from build123d import *

# Parameters (mm, degrees)
F0_W     = 64.5160431693
F0_H     = 21.2102837178
F1_DEPTH = 25.4
F3_DEPTH = 51.816
F5_DEPTH = 78.486
F6_DEPTH = 43.18


with BuildPart() as f1:
    # F0 (on Top) → F1 (new body)
    with BuildSketch(Plane.XY):
        with Locations((-13.5457146427, -10.1202105203)):
            Rectangle(F0_W, F0_H)
        with Locations((-13.5457146427, -31.3304942381)):
            Rectangle(F0_W, F0_H)
        Polygon((-56.0653362274, -41.935636097), (-45.8037362274, -41.935636097), (-45.8037362274, -20.7253523792), (-45.8037362274, 0.4849313386), (-56.0653362274, 0.4849313386), (-56.0653362274, -20.7253523792), align=None)
    extrude(amount=F1_DEPTH)

    # F2 (on face) → F3 (cut)
    with BuildSketch(Plane.XZ.offset(41.935636097)):
        with BuildLine():
            ThreePointArc((-44.145979319, 1.0321285638), (-44.1486688564, 1.034928695), (-44.1513573992, 1.0377297813))
            Line((-44.1513573992, 1.0377297813), (-45.9468774498, 1.1715529611))
            Line((-45.9468774498, 1.1715529611), (-44.145979319, 1.0321285638))
        make_face()
        with BuildLine():
            Line((-44.021862033, 16.3071069646), (-42.5827212101, 16.4143685911))
            ThreePointArc((-42.5827212101, 16.4143685911), (-42.5963025327, 16.4205333574), (-42.6111564435, 16.4218816897))
            Line((-42.6111564435, 16.4218816897), (-44.0158800553, 16.3131288738))
            ThreePointArc((-44.0158800553, 16.3131288738), (-44.0188716286, 16.3101184998), (-44.021862033, 16.3071069646))
        make_face()
        with BuildLine():
            Line((-45.9468774498, 16.1636322737), (-44.021862033, 16.3071069646))
            ThreePointArc((-44.021862033, 16.3071069646), (-44.0188716286, 16.3101184998), (-44.0158800553, 16.3131288738))
            Line((-44.0158800553, 16.3131288738), (-45.9468774498, 16.1636322737))
        make_face()
        with BuildLine():
            Line((7.372798217, 0), (-39.4825406605, 0))
            ThreePointArc((-39.4825406605, 0), (-38.9420590995, -0.1240575085), (-38.3949389733, -0.2144463942))
            Line((-38.3949389733, -0.2144463942), (7.372798217, -0.2144463942))
            Line((7.372798217, -0.2144463942), (7.372798217, 0))
        make_face()
        with BuildLine():
            ThreePointArc((-42.1654908366, 16.1326498601), (-40.5135421796, 16.9967749546), (-38.7185404025, 17.5003771437))
            Line((-38.7185404025, 17.5003771437), (-31.250141561, 17.5003771437))
            Line((-31.250141561, 17.5003771437), (-30.4561574012, 18.5174327344))
            Line((-30.4561574012, 18.5174327344), (-30.2798189223, 18.5174327344))
            Line((-30.2798189223, 18.5174327344), (-29.2510185391, 20.0290549546))
            Line((-29.2510185391, 20.0290549546), (-29.3390378356, 20.2990490943))
            Line((-29.3390378356, 20.2990490943), (-29.12097238, 20.5859038979))
            Line((-29.12097238, 20.5859038979), (-27.1381475031, 20.5859038979))
            Line((-27.1381475031, 20.5859038979), (-25.4679527134, 17.7082661539))
            Line((-25.4679527134, 17.7082661539), (-25.2317674458, 17.7082661539))
            Line((-25.2317674458, 17.7082661539), (-25.0472072512, 17.5003771437))
            Line((-25.0472072512, 17.5003771437), (-21.5065404773, 17.5003771437))
            Line((-21.5065404773, 17.5003771437), (-20.6615831703, 18.9307779074))
            Line((-20.6615831703, 18.9307779074), (-16.1240063608, 18.9307779074))
            Line((-16.1240063608, 18.9307779074), (-15.6271327287, 18.0392824113))
            Line((-15.6271327287, 18.0392824113), (-9.1119576246, 18.0392824113))
            Line((-9.1119576246, 18.0392824113), (-8.7532978505, 17.5003771437))
            Line((-8.7532978505, 17.5003771437), (0.1143061163, 17.5003771437))
            Line((0.1143061163, 17.5003771437), (0.7239317638, 17.9214961827))
            Line((0.7239317638, 17.9214961827), (2.5316779502, 17.9214961827))
            Line((2.5316779502, 17.9214961827), (3.1462397892, 17.5003771437))
            Line((3.1462397892, 17.5003771437), (13.8490989856, 17.5003771437))
            Line((13.8490989856, 17.5003771437), (17.7825259097, 2.6434083702))
            Line((17.7825259097, 2.6434083702), (17.0111356355, 1.5585501678))
            Line((17.0111356355, 1.5585501678), (7.372798217, 0.6550194812))
            Line((7.372798217, 0.6550194812), (7.372798217, 0))
            Line((7.372798217, 0), (18.7123069419, 0))
            Line((18.7123069419, 0), (18.7123069419, 25.4))
            Line((18.7123069419, 25.4), (-56.0653362274, 25.4))
            Line((-56.0653362274, 25.4), (-56.0653362274, 0))
            Line((-56.0653362274, 0), (-39.4825406605, 0))
            ThreePointArc((-39.4825406605, 0), (-40.8736718435, 0.4904810681), (-42.1654908366, 1.2025353747))
            Line((-42.1654908366, 1.2025353747), (-42.5827212101, 0.9208166436))
            Line((-42.5827212101, 0.9208166436), (-44.1513573992, 1.0377297813))
            ThreePointArc((-44.1513573992, 1.0377297813), (-44.1486688564, 1.034928695), (-44.145979319, 1.0321285638))
            Line((-44.145979319, 1.0321285638), (-45.9468774498, 1.1715529611))
            Line((-45.9468774498, 1.1715529611), (-46.4343652129, 1.4113573482))
            Line((-46.4343652129, 1.4113573482), (-49.6125221252, 4.1695129251))
            Line((-49.6125221252, 4.1695129251), (-55.1616996527, 5.3079299753))
            Line((-55.1616996527, 5.3079299753), (-55.7882027962, 5.8516391712))
            Line((-55.7882027962, 5.8516391712), (-55.7882027962, 8.6675926174))
            Line((-55.7882027962, 8.6675926174), (-55.7882027962, 11.4835460635))
            Line((-55.7882027962, 11.4835460635), (-55.1616996527, 12.0272552595))
            Line((-55.1616996527, 12.0272552595), (-49.6125221252, 13.1656723097))
            Line((-49.6125221252, 13.1656723097), (-46.4343652129, 15.9238278866))
            Line((-46.4343652129, 15.9238278866), (-45.9468774498, 16.1636322737))
            Line((-45.9468774498, 16.1636322737), (-44.0158800553, 16.3131288738))
            Line((-44.0158800553, 16.3131288738), (-42.6111564435, 16.4218816897))
            ThreePointArc((-42.6111564435, 16.4218816897), (-42.5963025327, 16.4205333574), (-42.5827212101, 16.4143685911))
            Line((-42.5827212101, 16.4143685911), (-42.1654908366, 16.1326498601))
        make_face()
    extrude(amount=-F3_DEPTH, mode=Mode.SUBTRACT)

    # F4 (on Right) → F5 (cut)
    with BuildSketch(Plane.YZ):
        Polygon((-9.7505459562, 19.0722569823), (-8.6611686274, 17.2283314168), (-8.1623115887, 17.2283314168), (0.8263854931, 1.7911824398), (1.259337645, 21.2465394288), (-42.2770902514, 21.2465394288), (-42.2770902514, 1.7911824398), (-33.2883931696, 17.2283314168), (-31.1412010342, 17.2283314168), (-30.3681883961, 18.0637445301), (-30.1878191531, 18.0637445301), (-28.7448633462, 20.6411108375), (-26.786563918, 20.6411108375), (-25.3436081111, 18.2183869183), (-24.0552537143, 18.2183869183), (-23.4626121819, 17.5740458071), (-22.3917532712, 17.5740458071), (-21.7214301229, 17.9864261299), (-19.8657140136, 17.9864261299), (-19.1957950592, 17.5740458071), (-18.0102344602, 17.5740458071), (-17.4616630302, 18.078601868), (-14.4639806944, 18.078601868), (-14.4639806944, 18.8015084714), (-14.2472516745, 19.0722569823), align=None)
    extrude(amount=-F5_DEPTH, mode=Mode.SUBTRACT)

    # F4 (on Right) → F6 (cut)
    with BuildSketch(Plane.YZ):
        Polygon((-9.7505459562, 19.0722569823), (-8.6611686274, 17.2283314168), (-8.1623115887, 17.2283314168), (0.8263854931, 1.7911824398), (1.259337645, 21.2465394288), (-42.2770902514, 21.2465394288), (-42.2770902514, 1.7911824398), (-33.2883931696, 17.2283314168), (-31.1412010342, 17.2283314168), (-30.3681883961, 18.0637445301), (-30.1878191531, 18.0637445301), (-28.7448633462, 20.6411108375), (-26.786563918, 20.6411108375), (-25.3436081111, 18.2183869183), (-24.0552537143, 18.2183869183), (-23.4626121819, 17.5740458071), (-22.3917532712, 17.5740458071), (-21.7214301229, 17.9864261299), (-19.8657140136, 17.9864261299), (-19.1957950592, 17.5740458071), (-18.0102344602, 17.5740458071), (-17.4616630302, 18.078601868), (-14.4639806944, 18.078601868), (-14.4639806944, 18.8015084714), (-14.2472516745, 19.0722569823), align=None)
    extrude(amount=F6_DEPTH, mode=Mode.SUBTRACT)


solid = f1.part
For this review, take the finished solid that the model builds, in its own axes (mm). A direction names the side the tool comes from. Round coordinates to 2 decimals unless told otherwise and drop trailing zeros. Loops run counter-clockwise (first coordinate to the right, second up) from the corner with the lowest first, then second, coordinate; pieces in that order, holes last. Notation, with made-up numbers: (64, 6) - (106, 6) arc R19 cw to (106, 24) - close; hole circle Ø3 at (89, 2.25). An arc over 180 degrees is marked (long way). Put each result on its own line as item: value. Start each with the question number.
1. Consider section A-A on x = -14. State the section outline as (y, z) points, plus the area to 3 significant figures.
2. For probe 1 along X at (y, z) = (-30, 18.25); probe 2 along Z at (x, y) = (-7, -8.5); probe 3 along Y at (x, z) = (-4, 8.5), list the stretches that pass through material, from the lowest coordinate up. Write a range as [from, to].
3. Consider section C-C on x = -37.5. State the section outline as (y, z) points, plus the area to 3 significant figures.
4. For faces 1 (the flat face through (-17.1, -9, 17.8)), 2 (the flat face through (-15, -21, 17.986)), 3 (the cylindrical face through (-40.85, -21.02, 0.48)), 4 (the flat face through (-26.1, -27.2, 18.8)), 5 (the flat face through (-18, -12, 18.931)), list the 3-axis set-ups (+Z, -Z, +X, -X, +Y, -Y) from which the entire face can be reached by the end or side of a thin tool; tool diameter is ignored.
5. Mouldability with a two-part tool opening along Y and no side actions: class faces 6 (the flat face through (-15, 0.485, 1)), 7 (the flat face through (-28, -16, 18.079)), 8 (the flat face through (2, -21, 17.921)), 9 (the flat face through (-15, -41.936, 1)) as +Y half, -Y half, draft (parallel to the pull), parting line (faces both ways), or undercut.
6. Consider section D-D on z = 10.75. State the section outline as (x, y) points, plus the area to 3 significant figures.
7. Consider section B-B on y = -2.5. State the section outline as (x, z) points.
8. Insertion check: P1, Ø3, axis at x = -48, z = 6, coming from the +Y side; P2, Ø5, axis at x = -0.5, z = 6.5, coming from the -Y side; P3, Ø0.5, axis at x = 1.5, y = -26, coming from the +Z side. Each pin has a flat end and moves straight along its axis. Give the tip position at first contact, or say it passes through.
Result sheet:
1. outline: (-41.94, 0) - (0.48, 0) - (0.48, 2.38) - (-8.16, 17.23) - (-8.66, 17.23) - (-9.14, 18.04) - (-17.5, 18.04) - (-18.01, 17.57) - (-19.2, 17.57) - (-19.87, 17.99) - (-21.72, 17.99) - (-22.39, 17.57) - (-23.46, 17.57) - (-23.89, 18.04) - (-30.39, 18.04) - (-31.14, 17.23) - (-33.29, 17.23) - (-41.94, 2.38) - close
1. area: 618 mm^2
2. probe 1: [-30.66, -25.78], [-21.06, -15.74]
2. probe 2: [0, 17.23]
2. probe 3: [-38.37, -3.08]
3. outline: (-41.94, 0) - (0.48, 0) - (0.48, 2.38) - (-8.16, 17.23) - (-8.66, 17.23) - (-8.82, 17.5) - (-30.89, 17.5) - (-31.14, 17.23) - (-33.29, 17.23) - (-41.94, 2.38) - close
3. area: 608 mm^2
4. face 1: +Z, +X, -X, +Y
4. face 2: +Z, +X, -X
4. face 3: -Z, +Y, -Y
4. face 4: +Z, +Y, -Y
4. face 5: +Z, +X, +Y, -Y
5. face 6: +Y half
5. face 7: undercut
5. face 8: draft
5. face 9: -Y half
6. outline: (-55.79, -37.06) - (15.64, -37.06) - (15.64, -4.39) - (-55.79, -4.39) - close
6. area: 2,330 mm^2
7. outline: (-55.79, 5.85) - (-55.16, 5.31) - (-49.61, 4.17) - (-46.43, 1.41) - (-45.95, 1.17) - (-42.58, 0.92) - (-42.17, 1.2) arc R8.96 ccw to (-39.48, 0) - (7.37, 0) - (7.37, 0.66) - (17.01, 1.56) - (17.78, 2.64) - (16.5, 7.5) - (-55.79, 7.5) - close
8. P1: y = -0.75
8. P2: y = -40.99
8. P3: z = 17.92
